Verification items for the finished model (mm, model axes). Give positions to 0.01 mm unless a question says otherwise; leave off trailing zeros. Loops run counter-clockwise (first coordinate to the right, second up) from the corner with the lowest first, then second, coordinate; pieces in that order, holes last. Notation, with made-up numbers: M 30,31.25 L 76,31.25 A17 ccw 76,59.25 Z; hole C -5.75,37.25 d3. An arc over 180 degrees is marked long. Use CSV: the item, a comma, the result in double quotes.
from build123d import *

# Parameters (mm, degrees)
CUT_EXTRUDE1_START = -25.4
SKETCH2_W          = 6.35
SKETCH2_H          = 19.05
CUT_EXTRUDE1_DEPTH = 25.4


with BuildPart() as part:
    # Sketch1 → Revolve1 (revolve)
    with BuildSketch(Plane.XY):
        Polygon((528.662376284, -1604.36232837), (529.424259242, -1605.827024707), (323.502507791, -1712.940198389), (322.740624833, -1711.475502052), align=None)
    revolve(axis=Axis((319.107029188, -1704.490027216, 0), (0.887157078, 0.46146757, 0)))

    # Sketch2 → Cut-Extrude1 (cut)
    with BuildSketch(Plane(origin=(-240.734168067, -125.221355071, 0), x_dir=(0, 0, -1), z_dir=(0.887157078, 0.46146757, 0)).offset(CUT_EXTRUDE1_START)):
        with Locations((0, -1659.407938171)):
            Rectangle(SKETCH2_W, SKETCH2_H)
    extrude(amount=CUT_EXTRUDE1_DEPTH, mode=Mode.SUBTRACT)


solid = part.part
(1) Section check A-A on z = -5.75. Record the cut outline in (x, y).
Calculated:
outline,"M 315.6,-1697.75 L 316.62,-1699.72 L 522.55,-1592.6 L 521.52,-1590.64 Z; M 321.59,-1709.26 L 322.61,-1711.23 L 528.53,-1604.11 L 527.51,-1602.15 Z"
(2) Mould release check, pull along Z, two halves, no side actions. Record for faces 1 (the flat face through (510, -1596, -3.175)), 2 (the cylindrical face through (419.674, -1649.851, 9.298)), 3 (the flat face through (316.48, -1699.44, -5.69)), 4 (the flat face through (517, -1611, -3.175)): released by +Z, released by -Z, zero draft, split by the parting line, or undercut.
Calculated:
face 1,"undercut"
face 2,"split by the parting line"
face 3,"zero draft"
face 4,"undercut"
(3) Depth check by flat-ended pin: pin 1 Ø8 at (x, y) = (393, -1648.5) entering from +Z; pin 2 Ø8 at (y, z) = (-1643, 2.5) entering from -X; pin 3 Ø2 at (x, z) = (490, -2) entering from +Y; pin 4 Ø14.5 at (x, y) = (523, -1607.5) entering from +Z. Enter the tip coordinate at first touch or a pass-through.
Calculated:
pin 1,"passes through"
pin 2,"stops at x = 409.48"
pin 3,"stops at y = -1604.54"
pin 4,"stops at z = 9.49"
(4) Scan lines: L1, parallel to Y at x = 482, z = -1; L2, parallel to Y at x = 459.5, z = 3; L3, parallel to X at y = -1612.5, z = 2.25. Record each from-to range of solid material in increasing order. Write a range as from..to.
Calculated:
L1,"y = -1630.44..-1628.56, -1610.96..-1609.08"
L2,"y = -1641.65..-1639.67, -1623.26..-1621.27"
L3,"x = 475.9..479.6"
